Source: CAD feature listing. Evaluate the final solid. Frame: model axes, mm. Face numbers are marked on the shaded views. Round coordinates to 2 decimals unless told otherwise and drop trailing zeros. Write each question's results on one line, items separated by ' | '. Start each with the question number.
1. Contact query for flat-ended pins moving along their axis: pin 1 Ø2 at (x, z) = (-2.56, -4.87) entering from +Y; pin 2 Ø1.5 at (x, y) = (1.5, 1) entering from -Z; pin 3 Ø1.9 at (x, z) = (0, -5.5) entering from -Y. Output: stop coordinate, or through.
2. Section A-A on y = 4.75. Give the number of separate pieces and of enclosed holes in the cut face, and give its area (3 significant figures).
3. Ray query, line 1 (Z direction, x = 4.25, y = 3.5); line 2 (X direction, y = 6.5, z = -0.5); line 3 (X direction, y = 4.5, z = 1.75). Return the intervals inside material, ascending.
4. Draft query along X for the marked faces 1 and 2. Return one class per face: released by +X, released by -X, zero draft, split by the parting line, or undercut.
from build123d import *

# Parameters (mm, degrees)
SKETCH_1_R          = 9.2
SKETCH_1_R_2        = 0.75
EXTRUDE_1_DEPTH     = 7
SKETCH_2_W          = 1
SKETCH_2_H          = 0.798143387
CUT_EXTRUDE_1_DEPTH = 7.5
SKETCH_6_R          = 3.75
CUT_EXTRUDE_3_DEPTH = 5
SKETCH_7_R          = 1.2
CUT_EXTRUDE_4_DEPTH = 1


with BuildPart() as part:
    # 草图1 → 凸台-拉伸1 (new body)
    with BuildSketch(Plane(origin=(0, 0, 0), x_dir=(1, 0, 0), z_dir=(0, 1, 0))):
        with Locations(Location((0, 0, 0), (0, 0, 270))):
            Circle(SKETCH_1_R)
        with Locations(Location((0, 5.5, 0), (0, 0, 270))):
            Circle(SKETCH_1_R_2, mode=Mode.SUBTRACT)
        with Locations(Location((2.555977446, 4.870008141, 0), (0, 0, 270))):
            Circle(SKETCH_1_R_2, mode=Mode.SUBTRACT)
        with Locations(Location((4.526411262, 3.124356107, 0), (0, 0, 270))):
            Circle(SKETCH_1_R_2, mode=Mode.SUBTRACT)
        with Locations(Location((5.459898808, 0.662951741, 0), (0, 0, 270))):
            Circle(SKETCH_1_R_2, mode=Mode.SUBTRACT)
        with Locations(Location((5.142589335, -1.950326879, 0), (0, 0, 270))):
            Circle(SKETCH_1_R_2, mode=Mode.SUBTRACT)
        with Locations(Location((3.64717462, -4.116809115, 0), (0, 0, 270))):
            Circle(SKETCH_1_R_2, mode=Mode.SUBTRACT)
        with Locations(Location((1.316236154, -5.340179996, 0), (0, 0, 270))):
            Circle(SKETCH_1_R_2, mode=Mode.SUBTRACT)
        with Locations(Location((-1.316236154, -5.340179996, 0), (0, 0, 270))):
            Circle(SKETCH_1_R_2, mode=Mode.SUBTRACT)
        with Locations(Location((-3.64717462, -4.116809115, 0), (0, 0, 270))):
            Circle(SKETCH_1_R_2, mode=Mode.SUBTRACT)
        with Locations(Location((-5.142589335, -1.950326879, 0), (0, 0, 270))):
            Circle(SKETCH_1_R_2, mode=Mode.SUBTRACT)
        with Locations(Location((-5.459898808, 0.662951741, 0), (0, 0, 270))):
            Circle(SKETCH_1_R_2, mode=Mode.SUBTRACT)
        with Locations(Location((-4.526411262, 3.124356107, 0), (0, 0, 270))):
            Circle(SKETCH_1_R_2, mode=Mode.SUBTRACT)
        with Locations(Location((-2.555977446, 4.870008141, 0), (0, 0, 270))):
            Circle(SKETCH_1_R_2, mode=Mode.SUBTRACT)
    extrude(amount=EXTRUDE_1_DEPTH)

    # 草图2 → 切除-拉伸1 (cut)
    with BuildSketch(Plane(origin=(0, 7, 0), x_dir=(1, 0, 0), z_dir=(0, 1, 0))):
        with Locations((0, 8.899071694)):
            Rectangle(SKETCH_2_W, SKETCH_2_H)
    extrude(amount=-CUT_EXTRUDE_1_DEPTH, mode=Mode.SUBTRACT)

    # 草图5 → 切除-旋转1 (revolve, cut)
    with BuildSketch(Plane(origin=(0, 0, 0), x_dir=(0, 0, -1), z_dir=(1, 0, 0))):
        with BuildLine():
            Line((-6, 3), (0, 3))
            Line((0, 3), (0, 0))
            Line((0, 0), (-9, 0))
            add(Edge.make_bspline(
                [(-9, 0), (-8.384481944, 1.295897354), (-7.512154342, 2.632195528), (-6, 3)],
                knots=[0, 0, 0, 0, 1, 1, 1, 1], degree=3))
        make_face()
    revolve(axis=Axis((0, 3, 0), (0, -1, 0)), mode=Mode.SUBTRACT)

    # 草图6 → 切除-拉伸3 (cut)
    with BuildSketch(Plane(origin=(0, 7, 0), x_dir=(1, 0, 0), z_dir=(0, 1, 0))):
        with Locations(Location((0, 0, 0), (0, 0, 270))):
            Circle(SKETCH_6_R)
    extrude(amount=-CUT_EXTRUDE_3_DEPTH, mode=Mode.SUBTRACT)

    # 草图7 → 切除-拉伸4 (cut)
    with BuildSketch(Plane(origin=(0, 7, 0), x_dir=(1, 0, 0), z_dir=(0, 1, 0))):
        with Locations(Location((0, 5.5, 0), (0, 0, 270))):
            Circle(SKETCH_7_R)
        with Locations(Location((2.555977446, 4.870008141, 0), (0, 0, 270))):
            Circle(SKETCH_7_R)
        with Locations(Location((4.526411262, 3.124356107, 0), (0, 0, 270))):
            Circle(SKETCH_7_R)
        with Locations(Location((5.459898808, 0.662951741, 0), (0, 0, 270))):
            Circle(SKETCH_7_R)
        with Locations(Location((5.142589335, -1.950326879, 0), (0, 0, 270))):
            Circle(SKETCH_7_R)
        with Locations(Location((3.64717462, -4.116809115, 0), (0, 0, 270))):
            Circle(SKETCH_7_R)
        with Locations(Location((1.316236154, -5.340179996, 0), (0, 0, 270))):
            Circle(SKETCH_7_R)
        with Locations(Location((-1.316236154, -5.340179996, 0), (0, 0, 270))):
            Circle(SKETCH_7_R)
        with Locations(Location((-3.64717462, -4.116809115, 0), (0, 0, 270))):
            Circle(SKETCH_7_R)
        with Locations(Location((-5.142589335, -1.950326879, 0), (0, 0, 270))):
            Circle(SKETCH_7_R)
        with Locations(Location((-5.459898808, 0.662951741, 0), (0, 0, 270))):
            Circle(SKETCH_7_R)
        with Locations(Location((-4.526411262, 3.124356107, 0), (0, 0, 270))):
            Circle(SKETCH_7_R)
        with Locations(Location((-2.555977446, 4.870008141, 0), (0, 0, 270))):
            Circle(SKETCH_7_R)
    extrude(amount=-CUT_EXTRUDE_4_DEPTH, mode=Mode.SUBTRACT)


solid = part.part
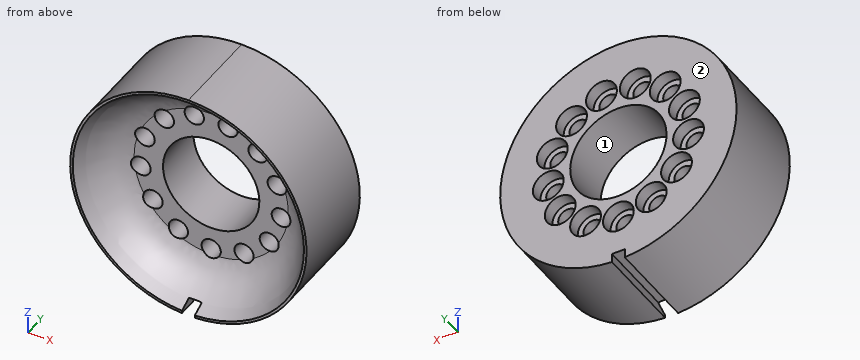
Taken from the geometry:
1) pin 1: y = 6 | pin 2: z = -9.17 | pin 3: y = 2.86
2) separate pieces: 1 | enclosed holes: 14 | area: 198 mm^2
3) line 1: -8.16 to -3.82, -2.43 to 3.67, 4.56 to 8.16 | line 2: -9.19 to -6.65, -4.27 to -3.72, 3.72 to 4.27, 6.65 to 9.19 | line 3: -9.03 to -5.87, -4.42 to -3.32, 3.32 to 4.42, 5.87 to 9.03
4) face 1: undercut | face 2: zero draft
